```python
from build123d import *

# Parameters (mm, degrees)
F0_R     = 2.15
F0_R_2   = 1.65
F1_DEPTH = 3


with BuildPart() as f1:
    # F0 (on Right) → F1 (new body)
    with BuildSketch(Plane.YZ):
        with BuildLine():
            Line((23.422032, 19.664407), (3.789993, 41.002941))
            ThreePointArc((3.789993, 41.002941), (0, 42.666043), (-3.789993, 41.002941))
            Line((-3.789993, 41.002941), (-23.422032, 19.664407))
            ThreePointArc((-23.422032, 19.664407), (-24.65, 16.516043), (-23.422032, 13.367679))
            Line((-23.422032, 13.367679), (-3.789993, -7.970854))
            ThreePointArc((-3.789993, -7.970854), (0, -9.633957), (3.789993, -7.970854))
            Line((3.789993, -7.970854), (23.422032, 13.367679))
            ThreePointArc((23.422032, 13.367679), (24.65, 16.516043), (23.422032, 19.664407))
        make_face()
        with Locations((0, -4.483957)):
            Circle(F0_R, mode=Mode.SUBTRACT)
        with Locations((-20, 16.516043)):
            Circle(F0_R_2, mode=Mode.SUBTRACT)
        with BuildLine():
            ThreePointArc((-13.75, 24.266043), (-13.164214, 25.680257), (-11.75, 26.266043))
            Line((-11.75, 26.266043), (11.75, 26.266043))
            ThreePointArc((11.75, 26.266043), (13.164214, 25.680257), (13.75, 24.266043))
            Line((13.75, 24.266043), (13.75, 8.766043))
            ThreePointArc((13.75, 8.766043), (13.164214, 7.35183), (11.75, 6.766043))
            Line((11.75, 6.766043), (-11.75, 6.766043))
            ThreePointArc((-11.75, 6.766043), (-13.164214, 7.35183), (-13.75, 8.766043))
            Line((-13.75, 8.766043), (-13.75, 24.266043))
        make_face(mode=Mode.SUBTRACT)
        with Locations((0, 37.516043)):
            Circle(F0_R, mode=Mode.SUBTRACT)
        with Locations((20, 16.516043)):
            Circle(F0_R_2, mode=Mode.SUBTRACT)
    extrude(amount=F1_DEPTH)


solid = f1.part
```
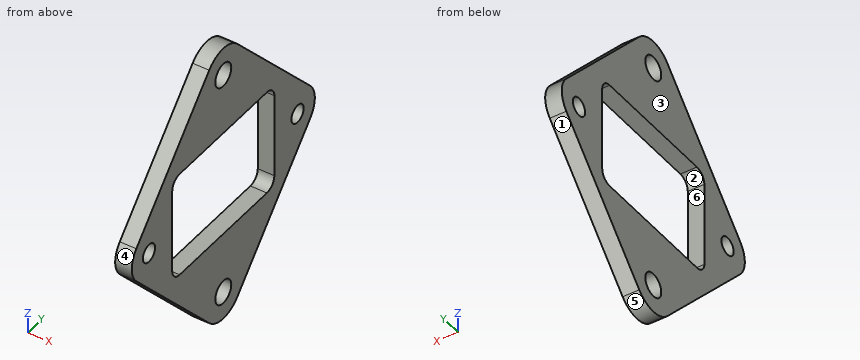
Work out the finished part from the listing and answer in its coordinate system (mm). Face numbers are marked on the shaded views. A direction names the side the tool comes from. Coordinates: 2 decimals unless noted, no trailing zeros. Loops run counter-clockwise (first coordinate to the right, second up) from the corner with the lowest first, then second, coordinate; pieces in that order, holes last.
1) Section D-D (y = -19.5) is taken. Give the vertices of the cut face in (x, z), plus the area to 3 significant figures.
Results:
outline: (0, 9.1) - (3, 9.1) - (3, 14.94) - (0, 14.94) - close; (0, 18.09) - (3, 18.09) - (3, 23.93) - (0, 23.93) - close
area: 35.0 mm2
2) Consider probe 1 along Z at (x, y) = (0.3, -0.5) (3 decimals); probe 2 along Z at (x, y) = (0.65, 1.5); probe 3 along Z at (x, y) = (1.5, -20). Determine where each line is inside the solid, lowest interval first.
Results:
probe 1: z = -9.61 to -6.575, -2.393 to 6.766, 26.266 to 35.425, 39.607 to 42.642
probe 2: z = -9.41 to -6.02, -2.94 to 6.77, 26.27 to 35.98, 39.06 to 42.44
probe 3: z = 9.65 to 14.87, 18.17 to 23.38
3) For the marked faces 5 and 6, determine the directions among +Z, -Z, +X, -X, +Y, -Y from which every point of the face is accessible in a straight line to the end or side of a thin tool.
Results:
face 5: -Z, +X, -X
face 6: +X, -X
4) Section B-B (z = -3) is taken. Give the vertices of the cut face in (x, y), plus the area to 3 significant figures.
Results:
outline: (0, -8.36) - (3, -8.36) - (3, -1.56) - (0, -1.56) - close; (0, 1.56) - (3, 1.56) - (3, 8.36) - (0, 8.36) - close
area: 40.8 mm2
5) Section A-A (y = 0) is taken. Give the vertices of the cut face in (x, z), plus the area to 3 significant figures.
Results:
outline: (0, -9.63) - (3, -9.63) - (3, -6.63) - (0, -6.63) - close; (0, -2.33) - (3, -2.33) - (3, 6.77) - (0, 6.77) - close; (0, 26.27) - (3, 26.27) - (3, 35.37) - (0, 35.37) - close; (0, 39.67) - (3, 39.67) - (3, 42.67) - (0, 42.67) - close
area: 72.6 mm2
6) A flat-ended cylindrical pin translates along its axis: pin 1 (1.5 mm diameter, centred on x = 0.5, y = -5.5, fed in from -Z). Find the tip coordinate at first contact, or state that the pin passes through.
Results:
pin 1: stops at z = -6.93
7) Section C-C (x = 0.5) is taken. Give the vertices of the cut face in (y, z), plus the area to 3 significant figures.
Results:
outline: (-23.42, 13.37) - (-3.79, -7.97) arc R5.15 ccw to (3.79, -7.97) - (23.42, 13.37) arc R4.65 ccw to (23.42, 19.66) - (3.79, 41) arc R5.15 ccw to (-3.79, 41) - (-23.42, 19.66) arc R4.65 ccw to start; hole circle Ø3.3 at (-20, 16.52); hole (-13.75, 8.77) arc R2 ccw to (-11.75, 6.77) - (11.75, 6.77) arc R2 ccw to (13.75, 8.77) - (13.75, 24.27) arc R2 ccw to (11.75, 26.27) - (-11.75, 26.27) arc R2 ccw to (-13.75, 24.27) - close; hole circle Ø4.3 at (0, -4.48); hole circle Ø4.3 at (0, 37.52); hole circle Ø3.3 at (20, 16.52)
area: 905 mm2
8) For a pull along Y with two mould halves and no side action, classify the marked faces 1, 2, 3 and 4 as +Y half, -Y half, draft (parallel to the pull), parting line (faces both ways), or undercut.
Results:
face 1: +Y half
face 2: undercut
face 3: draft
face 4: -Y half
